from build123d import *

# Parameters (mm, degrees)
F1_R     = 12
F2_DEPTH = 4
F3_DEPTH = 25
F4_W     = 2
F4_H     = 5.621666
F4_W_2   = 14.4
F4_H_2   = 10
F5_DEPTH = 4.001


with BuildPart() as f2:
    # F1 (on Front) → F2 (new body)
    with BuildSketch(Plane.XZ):
        Circle(F1_R)
    extrude(amount=-F2_DEPTH)

    # F0 (on Front) → F3 (join)
    with BuildSketch(Plane.XZ):
        Polygon((10.2, 0.4), (-10.2, 0.4), (-10.2, 2), (-11, 2), (-11, -2), (-10.2, -2), (-10.2, -0.4), (10.2, -0.4), (10.2, -2), (11, -2), (11, 2), (10.2, 2), align=None)
    extrude(amount=F3_DEPTH)

    # F4 (on face) → F5 (cut, through all)
    with BuildSketch(Plane.XZ):
        with Locations((0, 11.810833)):
            Rectangle(F4_W, F4_H)
        with Locations((0, -12.4)):
            Rectangle(F4_W_2, F4_H_2)
    extrude(amount=-F5_DEPTH, mode=Mode.SUBTRACT)


solid = f2.part
The listing builds one solid part. Answer for the finished solid, in the listing's coordinates (mm). A direction names the side the tool comes from. Round coordinates to 2 decimals unless told otherwise and drop trailing zeros. Order: outer loops, then holes, each group sorted by start corner. A loop starts at its lowest first (then second) coordinate and runs counter-clockwise, first axis right, second up. Notation, with made-up numbers: (47, 8.25) -> (55, 8.25) arc R17 cw to (55, 31.25) -> close; hole circle Ø11 at (83, -39). An arc over 180 degrees is marked (long way). One line per item, written item: value.
Item 1: For a pull along X with two mould halves and no side action, classify faces 1 (the flat face through (0, 4, 1)), 2 (the flat face through (-11, -12, 0)), 3 (the flat face through (0, 0, 1)) as released by +X, released by -X, zero draft, split by the parting line, or undercut.
Taken from the geometry:
face 1: zero draft
face 2: released by -X
face 3: undercut
Item 2: Find section C-C, the plane z = 9.5. Give the vertices of the cut face in (x, y).
Taken from the geometry:
outline: (-7.33, 0) -> (-1, 0) -> (-1, 4) -> (-7.33, 4) -> close; (1, 0) -> (7.33, 0) -> (7.33, 4) -> (1, 4) -> close
Item 3: Find section D-D, the plane y = -14.75. Give the vertices of the cut face in (x, z).
Taken from the geometry:
outline: (-11, -2) -> (-10.2, -2) -> (-10.2, -0.4) -> (10.2, -0.4) -> (10.2, -2) -> (11, -2) -> (11, 2) -> (10.2, 2) -> (10.2, 0.4) -> (-10.2, 0.4) -> (-10.2, 2) -> (-11, 2) -> close
Item 4: Given P1, Ø3, axis at x = 6.5, z = 9, coming from the -Y side; P2, Ø1.5, axis at x = -2, y = -4.5, coming from the +Z side; P3, Ø12, axis at y = -20.5, z = -4, coming from the +X side; P4, Ø5, axis at y = -4, z = 9, coming from the +X side, each flat-ended and moving along its own axis, determine where each tip first touches the part or whether it passes through.
Taken from the geometry:
P1: stops at y = 0
P2: stops at z = 0.4
P3: stops at x = 11
P4: passes through
Item 5: For faces 4 (the flat face through (10.6, -12.3, 2)), 5 (the flat face through (10.2, -12, -1)), 6 (the flat face through (1, 2, 10)), 7 (the flat face through (-10.2, -12, 1)), determine the directions among +Z, -Z, +X, -X, +Y, -Y from which every point of the face is accessible in a straight line to the end or side of a thin tool.
Taken from the geometry:
face 4: +Z, +X, -X, -Y
face 5: -Z, -Y
face 6: +Z, +Y, -Y
face 7: +Z, -Y
Item 6: Find section B-B, the plane z = 0. Give the vertices of the cut face in (x, y).
Taken from the geometry:
outline: (-12, 0) -> (-11, 0) -> (-11, -25) -> (11, -25) -> (11, 0) -> (12, 0) -> (12, 4) -> (-12, 4) -> close
Item 7: Find section A-A, the plane y = 0.75. Give the vertices of the cut face in (x, z).
Taken from the geometry:
outline: (-7.2, -9.6) -> (-7.2, -7.4) -> (7.2, -7.4) -> (7.2, -9.6) arc R12 ccw to (1, 11.96) -> (1, 9) -> (-1, 9) -> (-1, 11.96) arc R12 ccw to start
Item 8: Straight lines are drawn through the part: L1, parallel to X at y = -8.75, z = 0.5; L2, parallel to Y at x = -4.5, z = -0.75; L3, parallel to Z at x = -5.75, y = -23.75. For each, find the intervals that lie inside material, in ascending order.
Taken from the geometry:
L1: x = -11 to -10.2, 10.2 to 11
L2: y = 0 to 4
L3: z = -0.4 to 0.4
